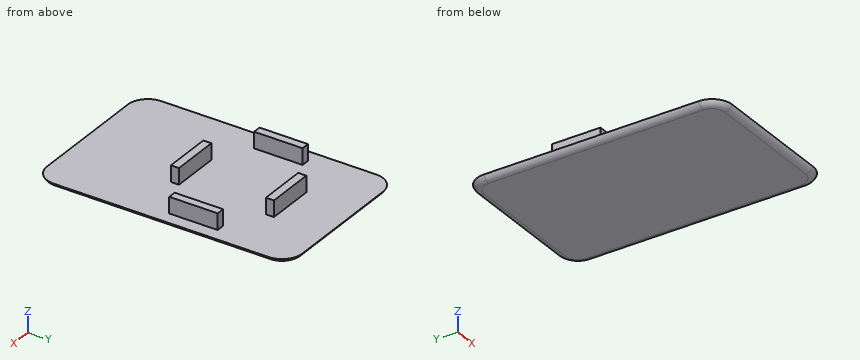
from build123d import *

# Parameters (mm, degrees)
SKETCH_1_W      = 39.94
SKETCH_1_H      = 63.19
EXTRUDE_1_DEPTH = 1.2
FILLET_1_R      = 5
FILLET_3_R      = 2
SKETCH_5_W      = 2
SKETCH_5_H      = 12
SKETCH_5_W_2    = 12
SKETCH_5_H_2    = 2
EXTRUDE_4_DEPTH = 4


with BuildPart() as part:
    # 草图1 → 凸台-拉伸1 (new body)
    with BuildSketch(Plane.XY):
        Rectangle(SKETCH_1_W, SKETCH_1_H)
    extrude(amount=EXTRUDE_1_DEPTH)

    # 圆角1
    fillet_1_edges = [part.edges().sort_by_distance(p)[0] for p in [
        (19.97, -31.595, 0.6),
        (-19.97, -31.595, 0.6),
        (-19.97, 31.595, 0.6),
        (19.97, 31.595, 0.6),
    ]]
    fillet(fillet_1_edges, radius=FILLET_1_R)

    # 圆角3
    # the kernel refuses this fillet: 2 mm, written as the material it takes off along each edge
    with BuildSketch(Plane(origin=(-14.97, -26.595, 0), x_dir=(0, -1, 0), z_dir=(1, 0, 0))) as fillet_3_piece_1:
        with BuildLine():
            CenterArc((3.166969722, -2), FILLET_3_R, 23.578178478, 66.421821522)
            Line((5, -1.2), (5.036660606, -1.184))
            ThreePointArc((5.036660606, -1.184), (5.04, -0.6), (5.04, 0))
            Line((5.04, 0), (5, 0.04))
            Line((5, 0.04), (3.166969722, 0.04))
            Line((3.166969722, 0.04), (3.166969722, 0))
        make_face()
    revolve(axis=Axis((-14.97, -26.595, 0), (0, 0, -1)), revolution_arc=90, mode=Mode.SUBTRACT)
    with BuildSketch(Plane(origin=(14.97, -31.595, 0), x_dir=(0, 1, 0), z_dir=(-1, 0, 0))) as fillet_3_piece_2:
        with BuildLine():
            CenterArc((1.833030278, -2), FILLET_3_R, 90, 66.421821522)
            Line((0, -1.2), (-0.036660606, -1.184))
            ThreePointArc((-0.036660606, -1.184), (-0.04, -0.6), (-0.04, 0))
            Line((-0.04, 0), (0, 0.04))
            Line((0, 0.04), (1.833030278, 0.04))
            Line((1.833030278, 0.04), (1.833030278, 0))
        make_face()
    extrude(amount=29.94, mode=Mode.SUBTRACT)
    with BuildSketch(Plane(origin=(14.97, -26.595, 0), x_dir=(1, 0, 0), z_dir=(0, 1, 0))) as fillet_3_piece_3:
        with BuildLine():
            CenterArc((3.166969722, -2), FILLET_3_R, 23.578178478, 66.421821522)
            Line((5, -1.2), (5.036660606, -1.184))
            ThreePointArc((5.036660606, -1.184), (5.04, -0.6), (5.04, 0))
            Line((5.04, 0), (5, 0.04))
            Line((5, 0.04), (3.166969722, 0.04))
            Line((3.166969722, 0.04), (3.166969722, 0))
        make_face()
    revolve(axis=Axis((14.97, -26.595, 0), (0, 0, -1)), revolution_arc=90, mode=Mode.SUBTRACT)
    with BuildSketch(Plane(origin=(19.97, 26.595, 0), x_dir=(-1, 0, 0), z_dir=(0, -1, 0)), Plane(origin=(-19.97, -26.595, 0), x_dir=(1, 0, 0), z_dir=(0, 1, 0))) as fillet_3_piece_4:
        with BuildLine():
            CenterArc((1.833030278, -2), FILLET_3_R, 90, 66.421821522)
            Line((0, -1.2), (-0.036660606, -1.184))
            ThreePointArc((-0.036660606, -1.184), (-0.04, -0.6), (-0.04, 0))
            Line((-0.04, 0), (0, 0.04))
            Line((0, 0.04), (1.833030278, 0.04))
            Line((1.833030278, 0.04), (1.833030278, 0))
        make_face()
    extrude(amount=53.19, mode=Mode.SUBTRACT)
    with BuildSketch(Plane(origin=(14.97, 26.595, 0), x_dir=(0, 1, 0), z_dir=(-1, 0, 0))) as fillet_3_piece_5:
        with BuildLine():
            CenterArc((3.166969722, -2), FILLET_3_R, 23.578178478, 66.421821522)
            Line((5, -1.2), (5.036660606, -1.184))
            ThreePointArc((5.036660606, -1.184), (5.04, -0.6), (5.04, 0))
            Line((5.04, 0), (5, 0.04))
            Line((5, 0.04), (3.166969722, 0.04))
            Line((3.166969722, 0.04), (3.166969722, 0))
        make_face()
    revolve(axis=Axis((14.97, 26.595, 0), (0, 0, -1)), revolution_arc=90, mode=Mode.SUBTRACT)
    with BuildSketch(Plane(origin=(-14.97, 31.595, 0), x_dir=(0, 0, 1), z_dir=(1, 0, 0))) as fillet_3_piece_6:
        with BuildLine():
            CenterArc((2, 1.833030278), FILLET_3_R, 180, 66.421821522)
            Line((0, 1.833030278), (-0.04, 1.833030278))
            Line((-0.04, 1.833030278), (-0.04, 0))
            Line((-0.04, 0), (0, -0.04))
            ThreePointArc((0, -0.04), (0.6, -0.04), (1.184, -0.036660606))
            Line((1.184, -0.036660606), (1.2, 0))
        make_face()
    extrude(amount=29.94, mode=Mode.SUBTRACT)
    with BuildSketch(Plane(origin=(-14.97, 26.595, 0), x_dir=(0, 1, 0), z_dir=(1, 0, 0))) as fillet_3_piece_7:
        with BuildLine():
            CenterArc((3.166969722, 2), FILLET_3_R, 270, 66.421821522)
            Line((5, 1.2), (5.036660606, 1.184))
            ThreePointArc((5.036660606, 1.184), (5.04, 0.6), (5.04, 0))
            Line((5.04, 0), (5, -0.04))
            Line((5, -0.04), (3.166969722, -0.04))
            Line((3.166969722, -0.04), (3.166969722, 0))
        make_face()
    revolve(axis=Axis((-14.97, 26.595, 0), (0, 0, 1)), revolution_arc=90, mode=Mode.SUBTRACT)

    # 草图5 → 凸台-拉伸4 (add)
    with BuildSketch(Plane.XY.offset(1.2)):
        with Locations((-15.75, 5.845)):
            Rectangle(SKETCH_5_W, SKETCH_5_H)
        with Locations((0, 17.595)):
            Rectangle(SKETCH_5_W_2, SKETCH_5_H_2)
        with Locations((0, -5.905)):
            Rectangle(SKETCH_5_W_2, SKETCH_5_H_2)
        with Locations((15.75, 5.845)):
            Rectangle(SKETCH_5_W, SKETCH_5_H)
    extrude(amount=EXTRUDE_4_DEPTH)


solid = part.part
Can you work these out from the model? Positions are in its coordinate system, mm. Round coordinates to 2 decimals unless told otherwise and drop trailing zeros. Write each loop counter-clockwise with the first axis right and the second up, starting at its lowest first coordinate (ties: lowest second). Pieces come first, ordered by that corner, then holes. Notation, with made-up numbers: (9, 71) - (67, 71) arc R17 cw to (67, 96) - close; hole circle Ø11 at (49.25, -10). An arc over 180 degrees is marked (long way). Write each question's results on one line, items separated by ' | '. Start each with the question number.
1) Suppose I cut it at C-C (y = 7.5). List the corners of the cut face in (x, z) for me, and give its area (3 significant figures).
2) For pin 1 Ø1.2 at (y, z) = (5, 3.5) entering from -X; pin 2 Ø1 at (x, z) = (15.5, 3) entering from -Y (3 decimals); pin 3 Ø3 at (y, z) = (9, 4) entering from +X, each with a flat end and sliding along its axis, tell me the tip position at first contact or that it passes through.
3) Suppose I cut it at A-A (z = 4.45). List the corners of the cut face in (x, y) for me (3 decimals), and give its area (3 significant figures).
4) Please list where these lines run through material, in increasing order: line 1 (Y direction, x = -4, z = 4.65) (3 decimals); line 2 (X direction, y = 2, z = 3.7); line 3 (Z direction, x = 9, y = 21.5).
5) Suppose I cut it at B-B (x = 4). List the corners of the cut face in (y, z) for me (3 decimals).
6) Suppose I cut it at D-D (y = 23). List the corners of the cut face in (x, z) for me.
Here are the results:
1) outline: (-19.97, 1.2) arc R2 ccw to (-18.14, 0) - (18.14, 0) arc R2 ccw to (19.97, 1.2) - (16.75, 1.2) - (16.75, 5.2) - (14.75, 5.2) - (14.75, 1.2) - (-14.75, 1.2) - (-14.75, 5.2) - (-16.75, 5.2) - (-16.75, 1.2) - close | area: 62.7 mm2
2) pin 1: stops at x = -16.75 | pin 2: stops at y = -0.155 | pin 3: stops at x = 16.75
3) outline: (-16.75, -0.155) - (-14.75, -0.155) - (-14.75, 11.845) - (-16.75, 11.845) - close; (-6, -6.905) - (6, -6.905) - (6, -4.905) - (-6, -4.905) - close; (-6, 16.595) - (6, 16.595) - (6, 18.595) - (-6, 18.595) - close; (14.75, -0.155) - (16.75, -0.155) - (16.75, 11.845) - (14.75, 11.845) - close | area: 96.0 mm2
4) line 1: y = -6.905 to -4.905, 16.595 to 18.595 | line 2: x = -16.75 to -14.75, 14.75 to 16.75 | line 3: z = 0 to 1.2
5) outline: (-31.595, 1.2) arc R2 ccw to (-29.762, 0) - (29.762, 0) arc R2 ccw to (31.595, 1.2) - (18.595, 1.2) - (18.595, 5.2) - (16.595, 5.2) - (16.595, 1.2) - (-4.905, 1.2) - (-4.905, 5.2) - (-6.905, 5.2) - (-6.905, 1.2) - close
6) outline: (-19.97, 1.2) arc R2 ccw to (-18.14, 0) - (18.14, 0) arc R2 ccw to (19.97, 1.2) - close
